```python
from build123d import *

# Parameters (mm, degrees)
F0_W     = 120
F0_H     = 200
F1_DEPTH = 100
F2_T     = -1
F3_R     = 1.5
F4_DEPTH = 130


with BuildPart() as f1:
    # F0 (on Top) → F1 (new body)
    with BuildSketch(Plane.XY):
        Rectangle(F0_W, F0_H)
    extrude(amount=F1_DEPTH)

    # F2
    f2_openings = [f1.faces().sort_by_distance(p)[0] for p in [
        (0, 0, 100),
    ]]
    offset(amount=F2_T, openings=f2_openings)

    # F3 (on face) → F4 (cut)
    with BuildSketch(Plane(origin=(-60, 0, 0), x_dir=(0, -1, 0), z_dir=(-1, 0, 0))):
        with Locations((0, 15)):
            Circle(F3_R)
    extrude(amount=-F4_DEPTH, mode=Mode.SUBTRACT)


solid = f1.part
```
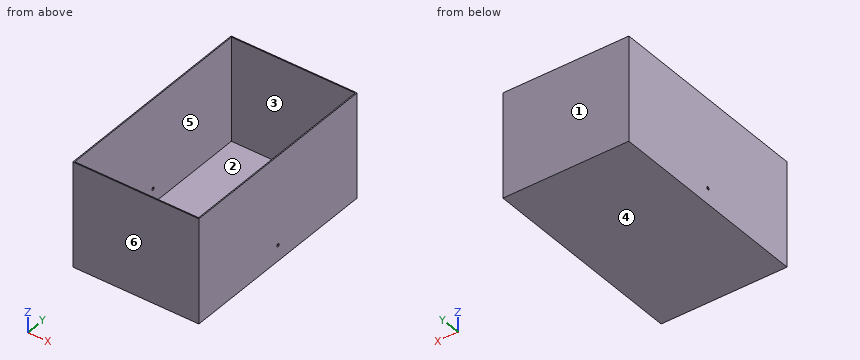
Build history of the part. All positions in model axes, mm. Face numbers are marked on the shaded views. A direction names the side the tool comes from. Give positions to 0.01 mm unless a question says otherwise; leave off trailing zeros. Loops run counter-clockwise (first coordinate to the right, second up) from the corner with the lowest first, then second, coordinate; pieces in that order, holes last.
Item 1: Slice it at A-A, the plane z = 24. List the corners of the cut face in (x, y), and give its area (3 significant figures).
Answers follow:
outline: (-60, -100) - (60, -100) - (60, 100) - (-60, 100) - close; hole (-59, -99) - (59, -99) - (59, 99) - (-59, 99) - close
area: 636 mm2
Item 2: Slice it at C-C, the plane x = 38.5. List the corners of the cut face in (y, z).
Answers follow:
outline: (-100, 0) - (100, 0) - (100, 100) - (99, 100) - (99, 1) - (-99, 1) - (-99, 100) - (-100, 100) - close
Item 3: Drill centre lines: line 1 (X direction, y = -60, z = 55); line 2 (Y direction, x = 3.5, z = 5.5); line 3 (Z direction, x = -59.65, y = 0). Where is each one in solid material? Low to high.
Answers follow:
line 1: x = -60 to -59, 59 to 60
line 2: y = -100 to -99, 99 to 100
line 3: z = 0 to 13.5, 16.5 to 100
Item 4: Pull direction Y, two halves, no side cores. Call the marked faces 1, 2, 3 and 4: released by +Y, released by -Y, zero draft, split by the parting line, or undercut.
Answers follow:
face 1: released by +Y
face 2: undercut
face 3: undercut
face 4: zero draft
Item 5: Which spindle directions (+Z, -Z, +X, -X, +Y, -Y) get a long thin tool onto all of the face, cutting with end or side? Do the marked faces 5 and 6. Say none if no direction does.
Answers follow:
face 5: +Z
face 6: +Z, -Z, +X, -X, -Y
Item 6: Slice it at B-B, the plane y = 87. List the corners of the cut face in (x, z), and give its area (3 significant figures).
Answers follow:
outline: (-60, 0) - (60, 0) - (60, 100) - (59, 100) - (59, 1) - (-59, 1) - (-59, 100) - (-60, 100) - close
area: 318 mm2
Item 7: Flat gauge pins, fed straight in: pin 1 (3 mm diameter, centred on x = 24, y = -67.5, fed in from -Z); pin 2 (2 mm diameter, centred on x = 40, y = -58, fed in from +Z). Where does each tip first touch, or does it go through?
Answers follow:
pin 1: stops at z = 0
pin 2: stops at z = 1
